Part model, mm, in its own coordinate system. A direction names the side the tool comes from. Give positions to 0.01 mm unless a question says otherwise; leave off trailing zeros. Order: outer loops, then holes, each group sorted by start corner. A loop starts at its lowest first (then second) coordinate and runs counter-clockwise, first axis right, second up. Notation, with made-up numbers: M 26,-33.5 L 52,-33.5 A18 ccw 52,-9.5 Z; hole C 44.5,27.25 d3. An arc over 180 degrees is marked long. Answer as a JSON object with one key per item and string values.
from build123d import *

# Parameters (mm, degrees)
F0_R     = 52
F0_R_2   = 50.5
F1_DEPTH = 15
F3_R     = 3.5
F4_DEPTH = 7
F5_R     = 1


with BuildPart() as f1:
    # F0 (on Top) → F1 (new body)
    with BuildSketch(Plane.XY):
        Circle(F0_R)
        Circle(F0_R_2, mode=Mode.SUBTRACT)
    extrude(amount=F1_DEPTH)

    # F3 (on offset) → F4 (join)
    with BuildSketch(Plane.YZ.offset(51.5)):
        with Locations((0, 7.729115)):
            Circle(F3_R)
    extrude(amount=F4_DEPTH)

    # F5
    f5_edges = [f1.edges().sort_by_distance(p)[0] for p in [
        (58.5, -3.5, 7.729115),
    ]]
    fillet(f5_edges, radius=F5_R)


solid = f1.part
1. Pin check, flat tips, straight feed: P1, Ø4, axis at x = 16, z = 9, coming from the +Y side; P2, Ø1, axis at y = -7.5, z = 5, coming from the -X side; P3, Ø6, axis at y = -32.5, z = 2.5, coming from the +X side. Stop position of each tip, or through.
Worked answers:
{"P1": "stops at y = 50.08", "P2": "stops at x = -51.53", "P3": "stops at x = 42.82"}
2. Cut at A-A on x = 0. Give the cut face in (y, z), plus the area to 3 significant figures.
Worked answers:
{"outline": "M -52,0 L -50.5,0 L -50.5,15 L -52,15 Z; M 50.5,0 L 52,0 L 52,15 L 50.5,15 Z", "area": "45.0 mm^2"}
3. Cut at B-B on y = 0. Give the cut face in (x, z), plus the area to 3 significant figures.
Worked answers:
{"outline": "M -52,0 L -50.5,0 L -50.5,15 L -52,15 Z; M 50.5,0 L 52,0 L 52,4.23 L 57.5,4.23 A1 ccw 58.5,5.23 L 58.5,10.23 A1 ccw 57.5,11.23 L 52,11.23 L 52,15 L 50.5,15 Z", "area": "90.1 mm^2"}
4. Probe line 1 along Y through (x, z) = (0, 10); line 2 along Y through (x, z) = (21.5, 9); line 3 along X through (y, z) = (-41, 14.5). List the from-to ranges inside material, lowest first.
Worked answers:
{"line 1": "y = -52 to -50.5, 50.5 to 52", "line 2": "y = -47.35 to -45.69, 45.69 to 47.35", "line 3": "x = -31.98 to -29.48, 29.48 to 31.98"}
5. Which spindle directions (+Z, -Z, +X, -X, +Y, -Y) get a long thin tool onto all of the face, cutting with end or side? Do faces 1 (the flat face through (-43, 27, 15)), 2 (the cylindrical face through (54.652, -0.759, 4.312)). Say none if no direction does.
Worked answers:
{"face 1": "+Z, +X, -X, +Y, -Y", "face 2": "+X"}
6. Two-plate mould, pull along X, no slides. Class faces 3 (the cylindrical face through (-10.95, -49.3, 7.4)), 4 (the flat face through (58.5, 0, 8)), 5 (the flat face through (-43, 27, 0)): +X half, -X half, draft (parallel to the pull), parting line (faces both ways), or undercut.
Worked answers:
{"face 3": "undercut", "face 4": "+X half", "face 5": "draft"}
7. Cut at C-C on z = 12.5. Give the cut face in (x, y), plus the area to 3 significant figures.
Worked answers:
{"outline": "C 0,0 d104; hole C 0,0 d101", "area": "483 mm^2"}
8. Cut at D-D on y = -41. Give the cut face in (x, z).
Worked answers:
{"outline": "M -31.98,0 L -29.48,0 L -29.48,15 L -31.98,15 Z; M 29.48,0 L 31.98,0 L 31.98,15 L 29.48,15 Z"}
